Autodesk Inventor part; units mm, degrees
ref_plane "YZ Plane" through (0, 0, 0) normal (1, 0, 0) x (0, 1, 0)
ref_plane "XZ Plane" through (0, 0, 0) normal (0, 1, 0) x (-1, 0, 0)
ref_plane "XY Plane" through (0, 0, 0) normal (0, 0, 1) x (1, 0, 0)
sketch "Esquisse1" plane through (0, 0, 0) normal (1, 0, 0) x (0, 1, 0)
  line L0 (7.5, 0) -> (138.9, 0)
  line L1 (146.4, -7.5) -> (146.4, -122.5)
  line L2 (138.9, -130) -> (7.5, -130)
  line L3 (0, -122.5) -> (0, -7.5)
  arc A0 (138.9, -130) -> (146.4, -122.5) centre (138.9, -122.5) ccw
  arc A1 (0, -122.5) -> (7.5, -130) centre (7.5, -122.5) ccw
  arc A2 (7.5, 0) -> (0, -7.5) centre (7.5, -7.5) ccw
  arc A3 (146.4, -7.5) -> (138.9, 0) centre (138.9, -7.5) ccw
  line L4 (15, -42.5) -> (131.4, -42.5)
  line L5 (131.4, -42.5) -> (131.4, -87.5)
  line L6 (131.4, -87.5) -> (15, -87.5)
  line L7 (15, -87.5) -> (15, -42.5)
  circle A4 centre (138.9, -122.5) radius 7.5
  line L8 (15, -42.5) -> (15, 0)
  line L9 (15, -87.5) -> (15, -130)
  line L10 (131.4, -87.5) -> (131.4, -130)
  line L11 (131.4, -42.5) -> (131.4, 0)
  circle A5 centre (7.5, -122.5) radius 7.5
  circle A6 centre (138.9, -7.5) radius 7.5
  circle A7 centre (7.5, -7.5) radius 7.5
  point P0 (0, 0)
  point P1 (146.4, -130)
  point P2 (146.4, 0)
  point P3 (0, -130)
  point P4 (73.2, -87.5)
  dimension "d0" = 146.4
  dimension "d1" = 130
  dimension "d2" = 7.5
  dimension "d3" = 7.5
  dimension "d4" = 116.4
  dimension "d5" = 45
  dimension "d11" = 42.5
  dimension "d12" = 42.5
  dimension "d13" = 15
  dimension "d104" = 131.4
  dimension "d107" = 115
sketch "Esquisse1 outline for Extrusion1" plane through (0, 0, 0) normal (1, 0, 0) x (0, 1, 0)
  line L0 (15, -87.5) -> (131.4, -87.5)
  line L1 (15, -130) -> (15, -87.5)
  line L2 (7.5, -130) -> (15, -130)
  arc A0 (0, -122.5) -> (7.5, -130) centre (7.5, -122.5) ccw
  line L3 (0, -7.5) -> (0, -122.5)
  arc A1 (7.5, 0) -> (0, -7.5) centre (7.5, -7.5) ccw
  line L4 (15, 0) -> (7.5, 0)
  line L5 (15, -42.5) -> (15, 0)
  line L6 (131.4, -42.5) -> (15, -42.5)
  line L7 (131.4, 0) -> (131.4, -42.5)
  line L8 (138.9, 0) -> (131.4, 0)
  arc A2 (146.4, -7.5) -> (138.9, 0) centre (138.9, -7.5) ccw
  line L9 (146.4, -122.5) -> (146.4, -7.5)
  arc A3 (138.9, -130) -> (146.4, -122.5) centre (138.9, -122.5) ccw
  line L10 (131.4, -130) -> (138.9, -130)
  line L11 (131.4, -87.5) -> (131.4, -130)
extrude "Extrusion1" add sketch "Esquisse1 outline for Extrusion1" along normal blind 7
sketch "Esquisse2" plane through (0, 0, 0) normal (-1, 0, 0) x (0, 0, 1)
  line L0 (-46.71, 27.48) -> (-83.29, 27.48)
  line L1 (-83.29, 27.48) -> (-83.29, 70.66)
  line L2 (-83.29, 70.66) -> (-46.71, 70.66)
  line L3 (-46.71, 70.66) -> (-46.71, 27.48)
  line L4 (-46.71, 75.74) -> (-83.29, 75.74)
  line L5 (-83.29, 75.74) -> (-83.29, 118.92)
  line L6 (-83.29, 118.92) -> (-46.71, 118.92)
  line L7 (-46.71, 118.92) -> (-46.71, 75.74)
  line L8 (-42.5, 131.4) -> (-42.5, 15)
  line L9 (-87.5, 15) -> (-87.5, 131.4)
  circle A0 centre (-83.29, 27.48) radius 2.3
  circle A1 centre (-46.71, 27.48) radius 2.3
  circle A2 centre (-46.71, 70.66) radius 2.3
  circle A3 centre (-83.29, 70.66) radius 2.3
  circle A4 centre (-83.29, 75.74) radius 2.3
  circle A5 centre (-46.71, 75.74) radius 2.3
  circle A6 centre (-46.71, 118.92) radius 2.3
  circle A7 centre (-83.29, 118.92) radius 2.3
  line L10 (-7.5, 0) -> (-122.5, 0)
  line L11 (-122.5, 146.4) -> (-7.5, 146.4)
  point P0 (0, 0)
  point P1 (-83.29, 49.07)
  dimension "d8" = 36.58
  dimension "d9" = 43.18
  dimension "d10" = 43.18
  dimension "d14" = 4.21
  dimension "d15" = 4.21
  dimension "d16" = 5.08
  dimension "d17" = 4.6
  dimension "d18" = 4.6
  dimension "d19" = 4.6
  dimension "d20" = 4.6
  dimension "d21" = 4.6
  dimension "d22" = 4.6
  dimension "d23" = 4.6
  dimension "d24" = 4.6
  dimension "d110" = 27.48
  dimension "d111" = 27.48
sketch "Esquisse2 outline for Extrusion2" plane through (0, 0, 0) normal (-1, 0, 0) x (0, 0, 1)
  circle A0 centre (-46.71, 118.92) radius 2.3
  circle A1 centre (-83.29, 118.92) radius 2.3
  circle A2 centre (-83.29, 75.74) radius 2.3
  circle A3 centre (-46.71, 75.74) radius 2.3
  circle A4 centre (-83.29, 70.66) radius 2.3
  circle A5 centre (-46.71, 70.66) radius 2.3
  circle A6 centre (-46.71, 27.48) radius 2.3
  circle A7 centre (-83.29, 27.48) radius 2.3
extrude "Extrusion2" cut sketch "Esquisse2 outline for Extrusion2" against normal blind 5.7
sketch "Esquisse3" plane through (0, 0, 0) normal (-1, 0, 0) x (0, 0, 1)
  arc A0 (-7.5, 0) -> (0, 7.5) centre (-7.5, 7.5) ccw
  circle A1 centre (-7.5, 7.5) radius 7.5
  arc A2 (-130, 7.5) -> (-122.5, 0) centre (-122.5, 7.5) ccw
  circle A3 centre (-122.5, 7.5) radius 7.5
  arc A4 (-122.5, 146.4) -> (-130, 138.9) centre (-122.5, 138.9) ccw
  circle A5 centre (-122.5, 138.9) radius 7.5
  arc A6 (0, 138.9) -> (-7.5, 146.4) centre (-7.5, 138.9) ccw
  circle A7 centre (-7.5, 138.9) radius 7.5
  point P0 (0, 0)
  point P1 (-7.5, 0)
  point P2 (-7.5, 146.4)
  point P3 (-130, 7.5)
sketch "Esquisse3 outline for Extrusion3" plane through (0, 0, 0) normal (-1, 0, 0) x (0, 0, 1)
  circle A0 centre (-7.5, 7.5) radius 7.5
  circle A1 centre (-7.5, 138.9) radius 7.5
  circle A2 centre (-122.5, 7.5) radius 7.5
  circle A3 centre (-122.5, 138.9) radius 7.5
extrude "Extrusion3" add sketch "Esquisse3 outline for Extrusion3" along normal blind 10
fillet "Congé1" radius 7.5 4 edges at (3.5, 131.4, 0) (3.5, 15, 0) (3.5, 131.4, -130) (3.5, 15, -130)
hole "Perçage5" at (-10, 7.5, -7.5) direction (1, 0, 0) diameter 6.3 depth 10
hole "Perçage6" at (-10, 138.9, -7.5) direction (1, 0, 0) diameter 6.3 depth 10
hole "Perçage7" at (-10, 138.9, -122.5) direction (1, 0, 0) diameter 6.3 depth 10
hole "Perçage8" at (-10, 7.5, -122.5) direction (1, 0, 0) diameter 6.3 depth 10
properties part number "base"
Geometry: final body of the model. Coordinates: model frame, mm. A direction names the side the tool comes from. Coordinates: 2 decimals unless noted, no trailing zeros. Order: outer loops, then holes, each group sorted by start corner. A loop starts at its lowest first (then second) coordinate and runs counter-clockwise, first axis right, second up. Notation, with made-up numbers: (-13, -32) -> (38, -32) arc R13 ccw to (38, -20) -> close; hole circle Ø3 at (-1, 86.5). An arc over 180 degrees is marked (long way). Answer in a Markdown table with one row per item.
Item 1: Ray query, L1, parallel to Y at x = 2.05, z = -83.29; L2, parallel to Z at x = -3.75, y = 7.5; L3, parallel to Y at x = -4.25, z = -7.5. Return the intervals inside material, ascending.
Return value:
| item | result |
|---|---|
| L1 | y = 0 to 25.18, 29.78 to 68.36, 72.96 to 73.44, 78.04 to 116.62, 121.22 to 146.4 |
| L2 | z = -130 to -125.65, -119.35 to -115, -15 to -10.65, -4.35 to 0 |
| L3 | y = 0 to 4.35, 10.65 to 15, 131.4 to 135.75, 142.05 to 146.4 |
Item 2: Access query for faces 1 (the flat face through (5.7, 76, -83)), 2 (the flat face through (-10, 8, -119)), 3 (the flat face through (3, 74, -42.5)). Directions: +Z, -Z, +X, -X, +Y, -Y. A direction counts if a zero-diameter tool reaches every point of the face in a straight line with its end or side. Return the directions, or none.
Return value:
| item | result |
|---|---|
| face 1 | -X |
| face 2 | +Z, -Z, -X, +Y, -Y |
| face 3 | +Z, +X, -X |
Item 3: Section A-A on x = -7.25. Output: boundary loops of the cut face in (y, z).
Return value:
| item | result |
|---|---|
| outline | circle Ø15 at (7.5, -122.5); circle Ø15 at (7.5, -7.5); circle Ø15 at (138.9, -122.5); circle Ø15 at (138.9, -7.5); hole circle Ø6.3 at (7.5, -122.5); hole circle Ø6.3 at (7.5, -7.5); hole circle Ø6.3 at (138.9, -122.5); hole circle Ø6.3 at (138.9, -7.5) |
Item 4: Section D-D on y = 75.74. Output: boundary loops of the cut face in (x, z), plus the area to 3 significant figures.
Return value:
| item | result |
|---|---|
| outline | (0, -87.5) -> (7, -87.5) -> (7, -42.5) -> (0, -42.5) -> (0, -44.41) -> (5.7, -44.41) -> (5.7, -49.01) -> (0, -49.01) -> (0, -80.99) -> (5.7, -80.99) -> (5.7, -85.59) -> (0, -85.59) -> close |
| area | 263 mm² |
Item 5: Draft query along Y for faces 4 (the flat face through (3, 146.4, -66)), 5 (the flat face through (3, 131.4, -25)), 6 (the flat face through (3, 0, -64)). Return one class per face: released by +Y, released by -Y, zero draft, split by the parting line, or undercut.
Return value:
| item | result |
|---|---|
| face 4 | released by +Y |
| face 5 | undercut |
| face 6 | released by -Y |
Item 6: Contact query for flat-ended pins moving along their axis: P1, Ø6, axis at y = 70.66, z = -46.71, coming from the -X side; P2, Ø10, axis at x = -7, z = -112.5, coming from the +Y side; P3, Ø2, axis at x = 5, y = 46.5, coming from the -Z side. Output: stop coordinate, or through.
Return value:
| item | result |
|---|---|
| P1 | stops at x = 0 |
| P2 | stops at y = 144.49 |
| P3 | stops at z = -87.5 |
Item 7: Section C-C on x = 3.75. State how many separate pieces and enclosed holes the cut face has, plus the area to 3 significant figures.
Return value:
| item | result |
|---|---|
| separate pieces | 1 |
| enclosed holes | 8 |
| area | 8,910 mm² |
Item 8: Section B-B on z = -38. Output: boundary loops of the cut face in (x, y).
Return value:
| item | result |
|---|---|
| outline | (0, 0) -> (7, 0) -> (7, 15) -> (0, 15) -> close; (0, 131.4) -> (7, 131.4) -> (7, 146.4) -> (0, 146.4) -> close |
